Here's how the part is built. I have some questions about the finished solid (model axes, mm). Face numbers are marked on the shaded views. A direction names the side the tool comes from. Coordinates: 2 decimals unless noted, no trailing zeros. Write each loop counter-clockwise with the first axis right and the second up, starting at its lowest first coordinate (ties: lowest second). Pieces come first, ordered by that corner, then holes. Notation, with made-up numbers: (78.5, -26.5) -> (103.5, -26.5) arc R24 cw to (103.5, -1.5) -> close; hole circle Ø1 at (83.5, -2). An arc over 180 degrees is marked (long way). Put each result on its own line as item: value. Start each with the question number.
Item 1: I need wall thicknesses on line 1 (Y direction, x = 20, z = 19); line 2 (Z direction, x = 0, y = -34); line 3 (Z direction, x = -1.5, y = -16). Which ranges of each line are inside material? Lowest first, please. Write a range as [from, to].
Item 2: On a 3-axis mill with a long thin cutter (end or side, diameter ignored), from which of +Z, -Z, +X, -X, +Y, -Y can I reach the whole of each face in a straight line? I mean the marked faces 1 and 2. Say none if no direction works.
Item 3: I want a section at B-B, the plane x = 0. List the corners of the cut face in (y, z) for me.
Item 4: I want a section at A-A, the plane z = 0. List the corners of the cut face in (x, y) for me.
Item 5: For pin 1 (1 mm diameter, centred on x = 17, y = -19, fed in from +Z); pin 2 (1 mm diameter, centred on x = -8, y = -29.5, fed in from -Z); pin 3 (1.5 mm diameter, centred on x = 1, y = -34, fed in from -Z), each with a flat end and sliding along its axis, tell me the tip position at first contact or that it passes through.
Item 6: I want a section at C-C, the plane y = -3. List the corners of the cut face in (x, z) for me, then the cut area to 3 significant figures.
Item 7: I want a section at D-D, the plane z = -23.5. List the corners of the cut face in (x, y) for me.
from build123d import *

# Parameters (mm, degrees)
F0_R     = 32.880177
F2_DEPTH = 25
F1_R     = 23.131498
F3_DEPTH = 15
F4_R     = 15.032714
F5_DEPTH = 15


with BuildPart() as f2:
    # F0 (on Front) → F2 (new body)
    with BuildSketch(Plane.XZ):
        Circle(F0_R)
    extrude(amount=F2_DEPTH)

    # F1 (on Front) → F3 (join)
    with BuildSketch(Plane.XZ):
        Circle(F1_R)
    extrude(amount=F3_DEPTH)

    # F4 (on face) → F5 (join)
    with BuildSketch(Plane.XZ.offset(25)):
        Circle(F4_R)
    extrude(amount=F5_DEPTH)


solid = f2.part
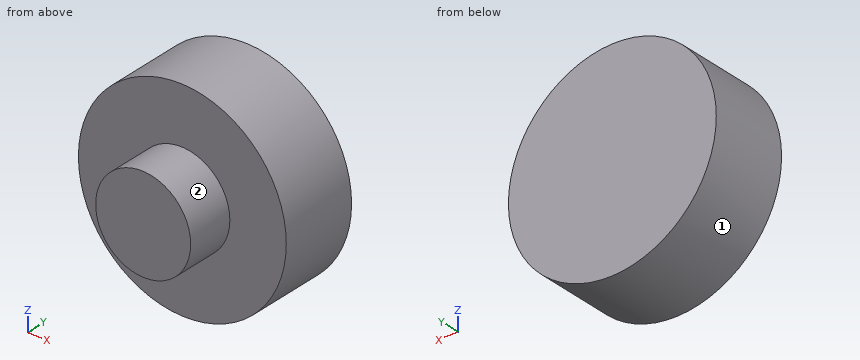
Calculated:
1. line 1: y = [-25, 0]
1. line 2: z = [-15.03, 15.03]
1. line 3: z = [-32.85, 32.85]
2. face 1: +Y, -Y
2. face 2: -Y
3. outline: (-40, -15.03) -> (-25, -15.03) -> (-25, -32.88) -> (0, -32.88) -> (0, 32.88) -> (-25, 32.88) -> (-25, 15.03) -> (-40, 15.03) -> close
4. outline: (-32.88, -25) -> (-15.03, -25) -> (-15.03, -40) -> (15.03, -40) -> (15.03, -25) -> (32.88, -25) -> (32.88, 0) -> (-32.88, 0) -> close
5. pin 1: stops at z = 28.44
5. pin 2: stops at z = -13.03
5. pin 3: stops at z = -15.03
6. outline: circle Ø65.76 at (0, 0)
6. area: 3,400 mm2
7. outline: (-23, -25) -> (23, -25) -> (23, 0) -> (-23, 0) -> close
